```python
from build123d import *

# Parameters (mm, degrees)
SKETCH1_W                   = 52
SKETCH1_H                   = 60.4
BOSS_EXTRUDE1_DEPTH         = 5
M3_CLEARANCE_HOLE1_D        = 3.2
TAP_DRILL_FOR_M3X0_5_TAP1_D = 2.5
FILLET1_R                   = 1


with BuildPart() as part:
    # Sketch1 → Boss-Extrude1 (new body)
    with BuildSketch(Plane(origin=(0, 0, 0), x_dir=(1, 0, 0), z_dir=(0, 1, 0))):
        with Locations((5, 0)):
            Rectangle(SKETCH1_W, SKETCH1_H)
        with BuildLine():
            Line((-11, -1.5), (-11, 1.5))
            ThreePointArc((-11, 1.5), (0, 12.5), (11, 1.5))
            Line((11, 1.5), (11, -1.5))
            ThreePointArc((11, -1.5), (0, -12.5), (-11, -1.5))
        make_face(mode=Mode.SUBTRACT)
        with BuildLine():
            Line((-18.5, 14), (-18.5, 17))
            ThreePointArc((-18.5, 17), (-15.5, 20), (-12.5, 17))
            Line((-12.5, 17), (-12.5, 14))
            ThreePointArc((-12.5, 14), (-15.5, 11), (-18.5, 14))
        make_face(mode=Mode.SUBTRACT)
        with BuildLine():
            Line((12.5, 14), (12.5, 17))
            ThreePointArc((12.5, 17), (15.5, 20), (18.5, 17))
            Line((18.5, 17), (18.5, 14))
            ThreePointArc((18.5, 14), (15.5, 11), (12.5, 14))
        make_face(mode=Mode.SUBTRACT)
        with BuildLine():
            Line((12.5, -17), (12.5, -14))
            ThreePointArc((12.5, -14), (15.5, -11), (18.5, -14))
            Line((18.5, -14), (18.5, -17))
            ThreePointArc((18.5, -17), (15.5, -20), (12.5, -17))
        make_face(mode=Mode.SUBTRACT)
        with BuildLine():
            Line((-18.5, -17), (-18.5, -14))
            ThreePointArc((-18.5, -14), (-15.5, -11), (-12.5, -14))
            Line((-12.5, -14), (-12.5, -17))
            ThreePointArc((-12.5, -17), (-15.5, -20), (-18.5, -17))
        make_face(mode=Mode.SUBTRACT)
    extrude(amount=BOSS_EXTRUDE1_DEPTH)

    # M3 Clearance Hole1 (through all)
    with Locations(Plane(origin=(0, 5, 0), x_dir=(1, 0, 0), z_dir=(0, 1, 0))):
        with Locations((-18, -27.2), (28, -27.2), (28, 27.2), (-18, 27.2)):
            Hole(M3_CLEARANCE_HOLE1_D / 2)

    # Tap Drill for M3x0.5 Tap1 (through all)
    with Locations(Plane(origin=(0, 5, 0), x_dir=(1, 0, 0), z_dir=(0, 1, 0))):
        with Locations((26, 0), (0, 25.5), (0, -25.5)):
            Hole(TAP_DRILL_FOR_M3X0_5_TAP1_D / 2)

    # Fillet1
    fillet1_edges = [part.edges().sort_by_distance(p)[0] for p in [
        (-21, 2.5, -30.2),
        (31, 2.5, -30.2),
        (31, 2.5, 30.2),
        (-21, 2.5, 30.2),
    ]]
    fillet(fillet1_edges, radius=FILLET1_R)


solid = part.part
```
Geometry: final body of the model. Coordinates: model frame, mm. A direction names the side the tool comes from. Round coordinates to 2 decimals unless told otherwise and drop trailing zeros. Order: outer loops, then holes, each group sorted by start corner. A loop starts at its lowest first (then second) coordinate and runs counter-clockwise, first axis right, second up. Notation, with made-up numbers: M 33,-7 L 84,-7 A8 cw 84,-2 Z; hole C -15,17 d9. An arc over 180 degrees is marked long. Use one line per item in the form item = value. Start each with the question number.
Q1. Cut plane D-D (y = 1.45). Count the separate pieces of the cut face and the enclosed holes in it, and give its area (3 significant figures).
Q2. Mould query, pull axis X, two halves, no side actions, for faces 1 (the face through (10, 0, -7)), 2 (the face through (-21, 2, 0)), 3 (the face through (11, 2, 0)). Classes: +X half, -X half, draft (parallel to the pull), parting line (faces both ways), or undercut.
Q3. Cut plane B-B (z = -6). Return loops of the section in (x, y).
Q4. Material intervals for line 1 (X direction, y = 2.45, z = 16); line 2 (Z direction, x = 28, y = 2); line 3 (Z direction, x = 0, y = 3.1), sorted ascending. Write a range as [from, to].
Q5. Pin query (flat end, axial travel): pin 1 Ø5 at (x, z) = (20, 9.5) entering from -Y. Return the tip coordinate at first contact, or that it passes through.
Q6. Cut plane C-C (x = -7). Return loops of the section in (y, z), and give its area (3 significant figures).
Q7. Cut plane A-A (x = -15.5). Return loops of the section in (y, z), and give its area (3 significant figures).
Q8. Access query for faces 4 (the face through (5, 2, 30.2)), 5 (the face through (12.5, 2, 16)). Directions: +Z, -Z, +X, -X, +Y, -Y. A direction counts if a zero-diameter tool reaches every point of the face in a straight line with its end or side. Return the directions, or none.
Geometry results:
q1.separate_pieces = 1
q1.enclosed_holes = 12
q1.area = 2,460 mm^2
q2.face_1 = draft
q2.face_2 = -X half
q2.face_3 = undercut
q3.outline = M -21,0 L -10.04,0 L -10.04,5 L -21,5 Z; M 10.04,0 L 31,0 L 31,5 L 10.04,5 Z
q4.line_1 = [-21, -18.5], [-12.5, 12.5], [18.5, 31]
q4.line_2 = [-30.2, -28.8], [-25.6, 25.6], [28.8, 30.2]
q4.line_3 = [-30.2, -26.75], [-24.25, -12.5], [12.5, 24.25], [26.75, 30.2]
q5.pin_1 = 0
q6.outline = M 0,-30.2 L 5,-30.2 L 5,-9.99 L 0,-9.99 Z; M 0,9.99 L 5,9.99 L 5,30.2 L 0,30.2 Z
q6.area = 202 mm^2
q7.outline = M 0,-30.2 L 5,-30.2 L 5,-20 L 0,-20 Z; M 0,-11 L 5,-11 L 5,11 L 0,11 Z; M 0,20 L 5,20 L 5,30.2 L 0,30.2 Z
q7.area = 212 mm^2
q8.face_4 = +Z, +X, -X, +Y, -Y
q8.face_5 = +Y, -Y
